from build123d import *

# Parameters (mm, degrees)
SKETCH1_R           = 4.5
BOSS_EXTRUDE1_DEPTH = 3


with BuildPart() as part:
    # Sketch1 → Boss-Extrude1 (new body)
    with BuildSketch(Plane.XY):
        with BuildLine():
            ThreePointArc((-25.027731338, -5.77818799), (-21.380140782, -6.093283782), (-18, -7.5))
            Line((-18, -7.5), (18, -7.5))
            ThreePointArc((18, -7.5), (21.380140782, -6.093283782), (25.027731338, -5.77818799))
            ThreePointArc((25.027731338, -5.77818799), (25.839696877, -5.861423129), (26.644067797, -6))
            ThreePointArc((26.644067797, -6), (32.644067797, 0), (26.644067797, 6))
            ThreePointArc((26.644067797, 6), (25.734720833, 5.818198735), (24.813267337, 5.713857688))
            ThreePointArc((24.813267337, 5.713857688), (21.259366627, 6.045176449), (18, 7.5))
            Line((18, 7.5), (-18, 7.5))
            ThreePointArc((-18, 7.5), (-21.259366627, 6.045176449), (-24.813267337, 5.713857688))
            ThreePointArc((-24.813267337, 5.713857688), (-25.734720833, 5.818198735), (-26.644067797, 6))
            ThreePointArc((-26.644067797, 6), (-32.644067797, 0), (-26.644067797, -6))
            ThreePointArc((-26.644067797, -6), (-25.839696877, -5.861423129), (-25.027731338, -5.77818799))
        make_face()
        with Locations((-26.644067797, 0)):
            Circle(SKETCH1_R, mode=Mode.SUBTRACT)
        with Locations((26.644067797, 0)):
            Circle(SKETCH1_R, mode=Mode.SUBTRACT)
    extrude(amount=BOSS_EXTRUDE1_DEPTH)


solid = part.part
Verification items for the finished model (mm, model axes). Coordinates: 2 decimals unless noted, no trailing zeros. Order: outer loops, then holes, each group sorted by start corner. A loop starts at its lowest first (then second) coordinate and runs counter-clockwise, first axis right, second up. Notation, with made-up numbers: M 66.5,16 L 110.5,16 A13 ccw 110.5,28 Z; hole C 39.5,0.25 d1. An arc over 180 degrees is marked long. One line per item, written item: value. Start each with the question number.
Item 1: Sectioned sample at A-A on y = 0. Record the cut outline in (x, z), then the cut area to 3 significant figures.
Item 2: Sectioned sample at C-C on y = -2.75. Record the cut outline in (x, z), then the cut area to 3 significant figures.
Item 3: Thickness scan on probe 1 along X at (y, z) = (0.75, 0.85); probe 2 along X at (y, z) = (-1.5, 1.4); probe 3 along Y at (x, z) = (-30, 0.8). Record the ranges inside material, lowest first.
Item 4: Mould release check, pull along X, two halves, no side actions. Record for faces 1 (the cylindrical face through (-22.35, 1.35, 1.48)), 2 (the cylindrical face through (-32.643, 0.132, 1.479)), 3 (the cylindrical face through (32.643, -0.132, 1.479)): pulls with the +X half, pulls with the -X half, needs draft (parallel to the pull), parting line crosses it, or undercut.
Item 5: Sectioned sample at B-B on z = 0.7. Record the cut outline in (x, y).
Calculated:
1. outline: M -32.64,0 L -31.14,0 L -31.14,3 L -32.64,3 Z; M -22.14,0 L 22.14,0 L 22.14,3 L -22.14,3 Z; M 31.14,0 L 32.64,0 L 32.64,3 L 31.14,3 Z
1. area: 142 mm^2
2. outline: M -31.98,0 L -30.21,0 L -30.21,3 L -31.98,3 Z; M -23.08,0 L 23.08,0 L 23.08,3 L -23.08,3 Z; M 30.21,0 L 31.98,0 L 31.98,3 L 30.21,3 Z
2. area: 149 mm^2
3. probe 1: -32.6 to -31.08, -22.21 to 22.21, 31.08 to 32.6
3. probe 2: -32.45 to -30.89, -22.4 to 22.4, 30.89 to 32.45
3. probe 3: -4.97 to -3, 3 to 4.97
4. face 1: undercut
4. face 2: pulls with the -X half
4. face 3: pulls with the +X half
5. outline: M -26.64,-6 A11.93 cw -18,-7.5 L 18,-7.5 A11.93 cw 26.64,-6 A6 ccw 26.64,6 A10.97 cw 18,7.5 L -18,7.5 A10.97 cw -26.64,6 A6 ccw Z; hole C -26.64,0 d9; hole C 26.64,0 d9
